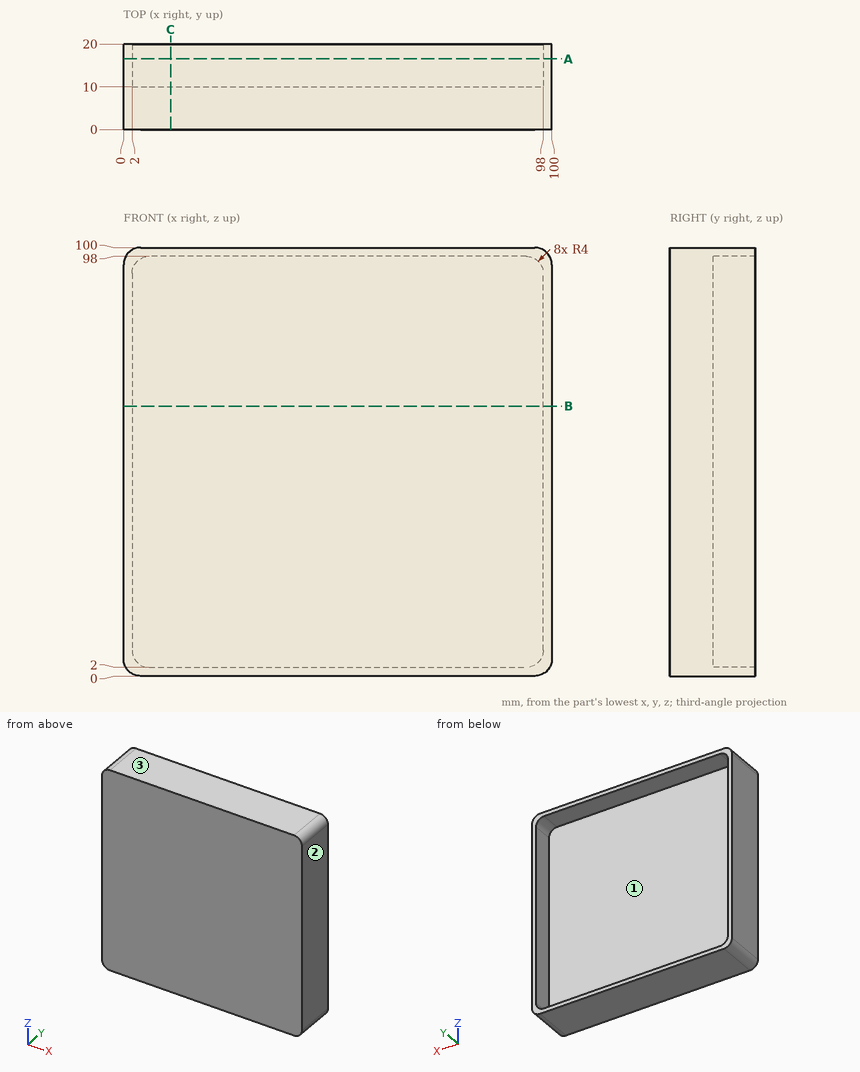
Could you check a few things on this drawing? It's one solid part, dimensions in mm from its lowest x, y, z. Give positions to 0.01 mm unless a question says otherwise; leave off trailing zeros. Loops run counter-clockwise (first coordinate to the right, second up) from the corner with the lowest first, then second, coordinate; pieces in that order, holes last. Notation, with made-up numbers: (44.5, -0.75) -> (102.5, -0.75) arc R33 cw to (102.5, 27.25) -> close; hole circle Ø7 at (-21.75, -15). An arc over 180 degrees is marked (long way). Answer as CSV lines item,"result". Start each with the question number.
(1) If we section it at B-B on z = 63: Write out the boundary of the cut face in (x, y).
(2) We'd pull the mould along X, two halves only. Please class the marked faces 1, 2 and 3: released by +X, released by -X, zero draft, split by the parting line, or undercut.
(3) If we section it at A-A on y = 16.5: Write out the boundary of the cut face in (x, z).
(4) I need wall thicknesses on probe 1 along X at (y, z) = (17.75, 71); probe 2 along Y at (x, z) = (92, 52). Which ranges of each line are inside material? Lowest first, please.
(5) If we section it at C-C on x = 11: Write out the boundary of the cut face in (y, z).
(6) I'm going to push flat-ended pins straight in: pin 1 Ø6 at (x, z) = (36.5, 11.5) entering from -Y; pin 2 Ø5 at (x, z) = (28, 76) entering from +Y. Where does each tip first touch, or does it pass through?
Computed:
1,outline,"(0, 0) -> (100, 0) -> (100, 20) -> (98, 20) -> (98, 10) -> (2, 10) -> (2, 20) -> (0, 20) -> close"
2,face 1,"undercut"
2,face 2,"released by +X"
2,face 3,"zero draft"
3,outline,"(0, 4) arc R4 ccw to (4, 0) -> (96, 0) arc R4 ccw to (100, 4) -> (100, 96) arc R4 ccw to (96, 100) -> (4, 100) arc R4 ccw to (0, 96) -> close; hole (2, 6) arc R4 ccw to (6, 2) -> (94, 2) arc R4 ccw to (98, 6) -> (98, 94) arc R4 ccw to (94, 98) -> (6, 98) arc R4 ccw to (2, 94) -> close"
4,probe 1,"x = 0 to 2, 98 to 100"
4,probe 2,"y = 0 to 10"
5,outline,"(0, 0) -> (20, 0) -> (20, 2) -> (10, 2) -> (10, 98) -> (20, 98) -> (20, 100) -> (0, 100) -> close"
6,pin 1,"stops at y = 0"
6,pin 2,"stops at y = 10"
